```python
from build123d import *

# Parameters (mm, degrees)
SKETCH1_R           = 15
BOSS_EXTRUDE1_DEPTH = 80
SKETCH2_W           = 8
SKETCH2_H           = 3.5
CUT_EXTRUDE2_DEPTH  = 83.764726786
SKETCH5_W           = 8.467594852
SKETCH5_H           = 0.933653361
CUT_EXTRUDE3_DEPTH  = 83.764726786


with BuildPart() as part:
    # Sketch1 → Boss-Extrude1 (new body)
    with BuildSketch(Plane(origin=(0, 0, 0), x_dir=(1, 0, 0), z_dir=(0, 1, 0))):
        with Locations(Location((0, 0, 0), (0, 0, 270))):
            Circle(SKETCH1_R)
    extrude(amount=BOSS_EXTRUDE1_DEPTH)

    # Sketch2 → Cut-Extrude2 (cut, through all)
    with BuildSketch(Plane(origin=(0, 80, 0), x_dir=(1, 0, 0), z_dir=(0, 1, 0))):
        with Locations((0, 12.706832295)):
            Rectangle(SKETCH2_W, SKETCH2_H)
    extrude(amount=-CUT_EXTRUDE2_DEPTH, mode=Mode.SUBTRACT)

    # Sketch5 → Cut-Extrude3 (cut, through all)
    with BuildSketch(Plane(origin=(0, 80, 0), x_dir=(1, 0, 0), z_dir=(0, 1, 0))):
        with Locations((0.233797426, 14.923658976)):
            Rectangle(SKETCH5_W, SKETCH5_H)
    extrude(amount=-CUT_EXTRUDE3_DEPTH, mode=Mode.SUBTRACT)


solid = part.part
```
Verification items for the finished model (mm, model axes). A direction names the side the tool comes from. Coordinates: 2 decimals unless noted, no trailing zeros. Loops run counter-clockwise (first coordinate to the right, second up) from the corner with the lowest first, then second, coordinate; pieces in that order, holes last. Notation, with made-up numbers: (-23, 45.5) - (18, 45.5) arc R34 ccw to (18, 77.5) - close; hole circle Ø5 at (-21.5, 85.25). An arc over 180 degrees is marked (long way). Answer as a JSON object with one key per item and string values.
(1) Cross-section at A-A, the plane x = -9. Record the boundary of the cut face in (y, z), then the cut area to 3 significant figures.
Response:
{"outline": "(0, -12) - (80, -12) - (80, 12) - (0, 12) - close", "area": "1,920 mm²"}
(2) Access from +Z, -Z, +X, -X, +Y, -Y to the whole of each face (thin tool, end or side, straight path). Record for faces 4 (the flat face through (0, 41, -10.957)), 5 (the flat face through (0, 0, 0)).
Response:
{"face 4": "-Z, +Y, -Y", "face 5": "+Z, -Z, +X, -X, -Y"}
(3) Cross-section at B-B, the plane y = 47.5. Record the boundary of the cut face in (x, z), then the cut area to 3 significant figures.
Response:
{"outline": "(-4, -14.46) - (-4, -10.96) - (4, -10.96) - (4, -14.46) arc R15 ccw (long way) to start", "area": "676 mm²"}
(4) Go/stop test with flat-tipped pins: pin 1 Ø1.5 at (x, y) = (2, 27.5) entering from -Z; pin 2 Ø4 at (x, y) = (-7.5, 53) entering from -Z; pin 3 Ø2 at (y, z) = (53.5, -10) entering from -X. Record where each tip stops, or that it passes through.
Response:
{"pin 1": "stops at z = -10.96", "pin 2": "stops at z = -13.96", "pin 3": "stops at x = -12"}
(5) Mould release check, pull along X, two halves, no side actions. Record for faces 1 (the cylindrical face through (-0.603, 39.44, 14.988)), 2 (the flat face through (0, 80, 0)), 3 (the flat face through (4, 41, -13)): pulls with the +X half, pulls with the -X half, needs draft (parallel to the pull), parting line crosses it, or undercut.
Response:
{"face 1": "parting line crosses it", "face 2": "needs draft", "face 3": "undercut"}
(6) Scan lines: line 1 along X through (y, z) = (12, -1); line 2 along Z through (x, y) = (1.5, 58.5); line 3 along Z through (x, y) = (9.5, 45.5). Record each from-to range of solid material in increasing order.
Response:
{"line 1": "x = -14.97 to 14.97", "line 2": "z = -10.96 to 14.92", "line 3": "z = -11.61 to 11.61"}
